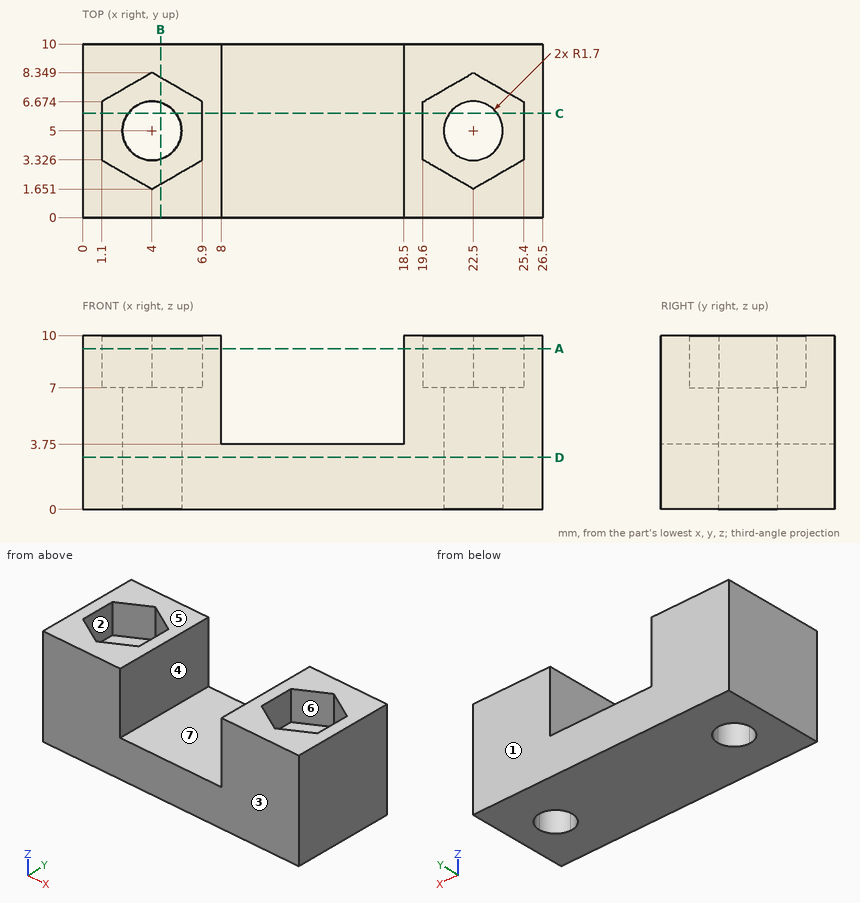
Could you check a few things on this drawing? It's one solid part, dimensions in mm from its lowest x, y, z. A direction names the side the tool comes from. Round coordinates to 2 decimals unless told otherwise and drop trailing zeros. Loops run counter-clockwise (first coordinate to the right, second up) from the corner with the lowest first, then second, coordinate; pieces in that order, holes last.
Q1. On a 3-axis mill with a long thin cutter (end or side, diameter ignored), from which of +Z, -Z, +X, -X, +Y, -Y can I reach the whole of each face in a straight line? I mean the marked faces 5, 6 and 7. Say none if no direction works.
Q2. I want a section at D-D (z = 3). Write out the boundary of the cut face in (x, y), and give its area (3 significant figures).
Q3. For P1, Ø1.7, axis at x = 24, y = 4.5, coming from the +Z side, with a flat end and sliding along its axis, tell me the tip position at first contact or that it passes through.
Q4. I want a section at C-C (y = 6). Give the number of separate pieces and of enclosed holes in the cut face, and give its area (3 significant figures).
Q5. I want a section at B-B (x = 4.5). Write out the boundary of the cut face in (y, z) (1 decimal).
Q6. Thinking about a two-plate mould opening in Y: for the marked faces 1, 2, 3 and 4, which applies, pulls with the +Y half, pulls with the -Y half, needs draft (parallel to the pull), parting line crosses it, or undercut?
Q7. I want a section at A-A (z = 9.25). Write out the boundary of the cut face in (x, y) (1 decimal).
Q8. Please list where these lines run through material, in increasing order: L1, parallel to X at y = 7, z = 5.75; L2, parallel to X at y = 4.5, z = 4.25 (1 decimal); L3, parallel to X at y = 4.75, z = 8.
Answer below:
1. face 5: +Z, +X, -X, +Y, -Y
1. face 6: +Z
1. face 7: +Z, +Y, -Y
2. outline: (0, 0) - (26.5, 0) - (26.5, 10) - (0, 10) - close; hole circle Ø3.4 at (4, 5); hole circle Ø3.4 at (22.5, 5)
2. area: 247 mm2
3. P1: stops at z = 7
4. separate pieces: 3
4. enclosed holes: 0
4. area: 126 mm2
5. outline: (0, 0) - (3.4, 0) - (3.4, 7) - (1.9, 7) - (1.9, 10) - (0, 10) - close; (6.6, 0) - (10, 0) - (10, 10) - (8.1, 10) - (8.1, 7) - (6.6, 7) - close
6. face 1: pulls with the +Y half
6. face 2: undercut
6. face 3: pulls with the -Y half
6. face 4: needs draft
7. outline: (0, 0) - (8, 0) - (8, 10) - (0, 10) - close; (18.5, 0) - (26.5, 0) - (26.5, 10) - (18.5, 10) - close; hole (1.1, 3.3) - (4, 1.7) - (6.9, 3.3) - (6.9, 6.7) - (4, 8.3) - (1.1, 6.7) - close; hole (19.6, 3.3) - (22.5, 1.7) - (25.4, 3.3) - (25.4, 6.7) - (22.5, 8.3) - (19.6, 6.7) - close
8. L1: x = 0 to 8, 18.5 to 26.5
8. L2: x = 0 to 2.4, 5.6 to 8, 18.5 to 20.9, 24.1 to 26.5
8. L3: x = 0 to 1.1, 6.9 to 8, 18.5 to 19.6, 25.4 to 26.5
